from build123d import *

# Parameters (mm, degrees)
SKETCH1_R           = 9
SKETCH1_R_2         = 3
BOSS_EXTRUDE1_DEPTH = 6
SKETCH2_R           = 7.25
SKETCH2_R_2         = 3
BOSS_EXTRUDE2_DEPTH = 11
SKETCH3_R           = 9
SKETCH3_R_2         = 3
BOSS_EXTRUDE3_DEPTH = 1
SKETCH4_R           = 1.5
CUT_EXTRUDE1_DEPTH  = 10
CUT_EXTRUDE4_START  = -1
SKETCH5_R           = 9
CUT_EXTRUDE4_DEPTH  = 11


with BuildPart() as part:
    # Sketch1 → Boss-Extrude1 (new body)
    with BuildSketch(Plane.XY):
        Circle(SKETCH1_R)
        Circle(SKETCH1_R_2, mode=Mode.SUBTRACT)
    extrude(amount=BOSS_EXTRUDE1_DEPTH)

    # Sketch2 → Boss-Extrude2 (add)
    with BuildSketch(Plane.XY.offset(6)):
        Circle(SKETCH2_R)
        Circle(SKETCH2_R_2, mode=Mode.SUBTRACT)
    extrude(amount=BOSS_EXTRUDE2_DEPTH)

    # Sketch3 → Boss-Extrude3 (add)
    with BuildSketch(Plane.XY.offset(17)):
        Circle(SKETCH3_R)
        Circle(SKETCH3_R_2, mode=Mode.SUBTRACT)
    extrude(amount=BOSS_EXTRUDE3_DEPTH)

    # Sketch4 → Cut-Extrude1 (cut, through all)
    with BuildSketch(Plane(origin=(0, 0, 0), x_dir=(1, 0, 0), z_dir=(0, 1, 0))):
        with Locations((0, -4)):
            Circle(SKETCH4_R)
    extrude(amount=-CUT_EXTRUDE1_DEPTH, mode=Mode.SUBTRACT)

    # Sketch5 → Cut-Extrude4 (cut)
    with BuildSketch(Plane.XY.offset(18).offset(CUT_EXTRUDE4_START)):
        Circle(SKETCH5_R)
        with BuildLine():
            Line((-0.95, 7.18748913), (-0.95, 6.92))
            ThreePointArc((-0.95, 6.92), (0, 5.97), (0.95, 6.92))
            Line((0.95, 6.92), (0.95, 7.18748913))
            ThreePointArc((0.95, 7.18748913), (1.414404835, 7.110693283), (1.872847455, 7.003923358))
            Line((1.872847455, 7.003923358), (1.770483796, 6.756795626))
            ThreePointArc((1.770483796, 6.756795626), (2.284620091, 5.515560809), (3.525854908, 6.029697104))
            Line((3.525854908, 6.029697104), (3.628218566, 6.276824837))
            ThreePointArc((3.628218566, 6.276824837), (4.027884188, 6.028154687), (4.410570862, 5.754073746))
            Line((4.410570862, 5.754073746), (4.221427484, 5.564930368))
            ThreePointArc((4.221427484, 5.564930368), (4.221427484, 4.221427484), (5.564930368, 4.221427484))
            Line((5.564930368, 4.221427484), (5.754073746, 4.410570862))
            ThreePointArc((5.754073746, 4.410570862), (6.028154689, 4.027884189), (6.276824837, 3.628218566))
            Line((6.276824837, 3.628218566), (6.029697104, 3.525854908))
            ThreePointArc((6.029697104, 3.525854908), (5.515560809, 2.284620091), (6.756795626, 1.770483796))
            Line((6.756795626, 1.770483796), (7.003923358, 1.872847455))
            ThreePointArc((7.003923358, 1.872847455), (7.110693283, 1.414404835), (7.18748913, 0.95))
            Line((7.18748913, 0.95), (6.92, 0.95))
            ThreePointArc((6.92, 0.95), (5.97, 0), (6.92, -0.95))
            Line((6.92, -0.95), (7.18748913, -0.95))
            ThreePointArc((7.18748913, -0.95), (7.110693283, -1.414404835), (7.003923358, -1.872847455))
            Line((7.003923358, -1.872847455), (6.756795626, -1.770483796))
            ThreePointArc((6.756795626, -1.770483796), (5.515560809, -2.284620091), (6.029697104, -3.525854908))
            Line((6.029697104, -3.525854908), (6.276824837, -3.628218566))
            ThreePointArc((6.276824837, -3.628218566), (6.028154689, -4.027884189), (5.754073746, -4.410570862))
            Line((5.754073746, -4.410570862), (5.564930368, -4.221427484))
            ThreePointArc((5.564930368, -4.221427484), (4.221427484, -4.221427484), (4.221427484, -5.564930368))
            Line((4.221427484, -5.564930368), (4.410570862, -5.754073746))
            ThreePointArc((4.410570862, -5.754073746), (4.027884189, -6.028154689), (3.628218566, -6.276824837))
            Line((3.628218566, -6.276824837), (3.525854908, -6.029697104))
            ThreePointArc((3.525854908, -6.029697104), (2.284620091, -5.515560809), (1.770483796, -6.756795626))
            Line((1.770483796, -6.756795626), (1.872847455, -7.003923358))
            ThreePointArc((1.872847455, -7.003923358), (1.414404835, -7.110693283), (0.95, -7.18748913))
            Line((0.95, -7.18748913), (0.95, -6.92))
            ThreePointArc((0.95, -6.92), (0, -5.97), (-0.95, -6.92))
            Line((-0.95, -6.92), (-0.95, -7.18748913))
            ThreePointArc((-0.95, -7.18748913), (-1.414404835, -7.110693283), (-1.872847455, -7.003923358))
            Line((-1.872847455, -7.003923358), (-1.770483796, -6.756795626))
            ThreePointArc((-1.770483796, -6.756795626), (-2.284620091, -5.515560809), (-3.525854908, -6.029697104))
            Line((-3.525854908, -6.029697104), (-3.628218566, -6.276824837))
            ThreePointArc((-3.628218566, -6.276824837), (-4.027884189, -6.028154689), (-4.410570862, -5.754073746))
            Line((-4.410570862, -5.754073746), (-4.221427484, -5.564930368))
            ThreePointArc((-4.221427484, -5.564930368), (-4.221427484, -4.221427484), (-5.564930368, -4.221427484))
            Line((-5.564930368, -4.221427484), (-5.754073746, -4.410570862))
            ThreePointArc((-5.754073746, -4.410570862), (-6.028154689, -4.027884189), (-6.276824837, -3.628218566))
            Line((-6.276824837, -3.628218566), (-6.029697104, -3.525854908))
            ThreePointArc((-6.029697104, -3.525854908), (-5.515560809, -2.284620091), (-6.756795626, -1.770483796))
            Line((-6.756795626, -1.770483796), (-7.003923358, -1.872847455))
            ThreePointArc((-7.003923358, -1.872847455), (-7.110693283, -1.414404835), (-7.18748913, -0.95))
            Line((-7.18748913, -0.95), (-6.92, -0.95))
            ThreePointArc((-6.92, -0.95), (-5.97, 0), (-6.92, 0.95))
            Line((-6.92, 0.95), (-7.18748913, 0.95))
            ThreePointArc((-7.18748913, 0.95), (-7.110693275, 1.414404833), (-7.003923358, 1.872847455))
            Line((-7.003923358, 1.872847455), (-6.756795626, 1.770483796))
            ThreePointArc((-6.756795626, 1.770483796), (-5.515560809, 2.284620091), (-6.029697104, 3.525854908))
            Line((-6.029697104, 3.525854908), (-6.276824837, 3.628218566))
            ThreePointArc((-6.276824837, 3.628218566), (-6.028154686, 4.027884187), (-5.754073746, 4.410570862))
            Line((-5.754073746, 4.410570862), (-5.564930368, 4.221427484))
            ThreePointArc((-5.564930368, 4.221427484), (-4.221427484, 4.221427484), (-4.221427484, 5.564930368))
            Line((-4.221427484, 5.564930368), (-4.410570862, 5.754073746))
            ThreePointArc((-4.410570862, 5.754073746), (-4.027884189, 6.028154689), (-3.628218566, 6.276824837))
            Line((-3.628218566, 6.276824837), (-3.525854908, 6.029697104))
            ThreePointArc((-3.525854908, 6.029697104), (-2.284620091, 5.515560809), (-1.770483796, 6.756795626))
            Line((-1.770483796, 6.756795626), (-1.872847455, 7.003923358))
            ThreePointArc((-1.872847455, 7.003923358), (-1.414404834, 7.11069328), (-0.95, 7.18748913))
        make_face(mode=Mode.SUBTRACT)
    extrude(amount=-CUT_EXTRUDE4_DEPTH, mode=Mode.SUBTRACT)


solid = part.part
Build history of the part. All positions in model axes, mm. A direction names the side the tool comes from. Give positions to 0.01 mm unless a question says otherwise; leave off trailing zeros. Loops run counter-clockwise (first coordinate to the right, second up) from the corner with the lowest first, then second, coordinate; pieces in that order, holes last. Notation, with made-up numbers: (87.25, 68) - (112.25, 68) arc R19 cw to (112.25, 77) - close; hole circle Ø7 at (87.25, 11.25). An arc over 180 degrees is marked (long way). Write item = value, one per line. Start each with the question number.
1) Band-saw the part on B-B on z = 1.5. Give the cut face in (x, y), plus the area to 3 significant figures.
2) Probe probe 1 along Z at (x, y) = (0, -7.5); probe 2 along Z at (x, y) = (4.75, -4); probe 3 along Y at (x, z) = (0, 13.25). List the from-to ranges inside material, lowest first. Write a range as from..to.
3) Band-saw the part on D-D on z = 4. Give the cut face in (x, y).
4) Tool access for faces 4 (the cylindrical face through (5.51, 2.3, 11.58)), 5 (the cylindrical face through (1.41, 7.11, 11.58)), 6 (the cylindrical face through (5.97, 0.02, 11.58)), 7 (the cylindrical face through (-1.41, -7.11, 11.58)), 8 (the cylindrical face through (-0.195, -5.756, 2.513)): list every direction of +Z, -Z, +X, -X, +Y, -Y with a clear straight run to the whole face (end or side of a thin tool).
5) Band-saw the part on A-A on y = 0. Give the cut face in (x, z).
6) Pull direction Y, two halves, no side cores. Call faces 1 (the cylindrical face through (-5.52, 2.27, 11.58)), 2 (the cylindrical face through (0.02, -5.97, 11.58)), 3 (the cylindrical face through (-7.11, 1.41, 11.58)): +Y half, -Y half, draft (parallel to the pull), parting line (faces both ways), or undercut.
7) Band-saw the part on C-C on y = -5. Give the cut face in (x, z).
8) Drop flat-ended pins along their axis: pin 1 Ø8 at (y, z) = (4.5, 2.5) entering from -X; pin 2 Ø3.5 at (x, y) = (0, 0) entering from +Z; pin 3 Ø1.5 at (x, z) = (0, 13.5) entering from +Y; pin 4 Ø4 at (x, z) = (7, 3.5) entering from -Y. Give the stop position or say it passes through.
Final values:
q1.outline = circle Ø18 at (0, 0); hole circle Ø6 at (0, 0)
q1.area = 226 mm²
q2.probe_1 = 0..2.5, 5.5..6, 17..18
q2.probe_2 = 0..6, 17..18
q2.probe_3 = -5.97..-3, 3..5.97
q3.outline = (-1.5, -8.87) - (-1.5, -2.6) arc R3 cw (long way) to (1.5, -2.6) - (1.5, -8.87) arc R9 ccw (long way) to start
q4.face_4 = none
q4.face_5 = +X, +Y
q4.face_6 = +X
q4.face_7 = -X, -Y
q4.face_8 = -Y
q5.outline = (-9, 0) - (-3, 0) - (-3, 18) - (-9, 18) - (-9, 17) - (-5.97, 17) - (-5.97, 6) - (-9, 6) - close; (3, 0) - (9, 0) - (9, 6) - (5.97, 6) - (5.97, 17) - (9, 17) - (9, 18) - (3, 18) - close
q6.face_1 = undercut
q6.face_2 = -Y half
q6.face_3 = +Y half
q7.outline = (-7.48, 0) - (7.48, 0) - (7.48, 6) - (3.95, 6) - (3.95, 17) - (7.48, 17) - (7.48, 18) - (-7.48, 18) - (-7.48, 17) - (-3.95, 17) - (-3.95, 6) - (-7.48, 6) - close; hole circle Ø3 at (0, 4)
q8.pin_1 = -8.99
q8.pin_2 = through
q8.pin_3 = 6.34
q8.pin_4 = -7.48
